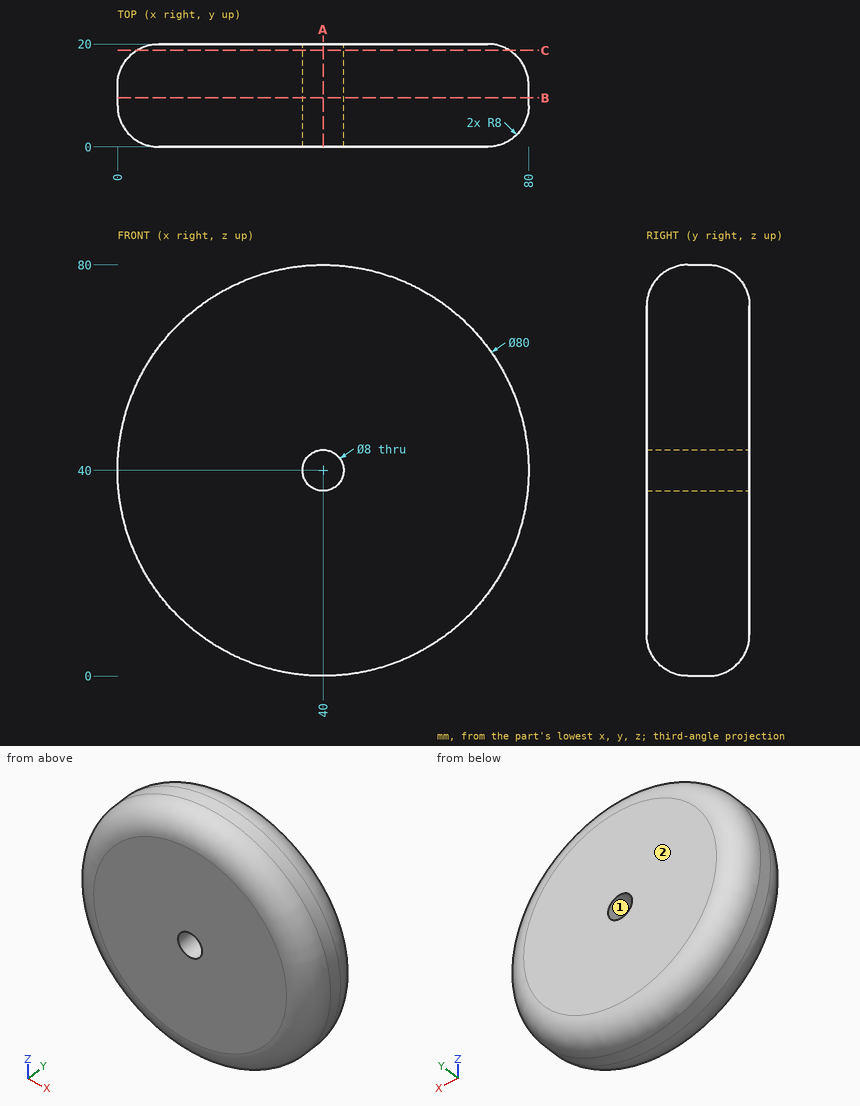
Geometry: see drawing. Coordinates: mm, zero at the bounding-box minimum. Round coordinates to 2 decimals unless told otherwise and drop trailing zeros. Loops run counter-clockwise (first coordinate to the right, second up) from the corner with the lowest first, then second, coordinate; pieces in that order, holes last. Notation, with made-up numbers: (-34.75, 55) -> (-27.75, 55) arc R22 ccw to (-27.75, 79) -> close; hole circle Ø10 at (64, 5.25). An arc over 180 degrees is marked (long way). Use one line per item in the form item = value. Start each with the question number.
Item 1: Material intervals for L1, parallel to Z at x = 40, y = 9.5; L2, parallel to X at y = 9, z = 64; L3, parallel to X at y = 13.75, z = 6.5, sorted ascending. Write a range as from..to.
Item 2: Section query C-C on y = 18.75. Return the cut outline in (x, z), then the cut area to 3 significant figures.
Item 3: Section query B-B on y = 9.5. Return the cut outline in (x, z), then the cut area to 3 significant figures.
Item 4: Section query A-A on x = 40. Return the cut outline in (y, z).
Item 5: Mould query, pull axis X, two halves, no side actions, for the marked faces 1 and 2. Classes: pulls with the +X half, pulls with the -X half, needs draft (parallel to the pull), parting line crosses it, or undercut.
Item 6: Contact query for flat-ended pins moving along their axis: pin 1 Ø8 at (x, y) = (59, 10.5) entering from +Z; pin 2 Ø5 at (x, y) = (14, 16) entering from -Z; pin 3 Ø1.5 at (y, z) = (5.5, 18) entering from -X. Output: stop coordinate, or through.
Ans:
q1.L1 = 0..36, 44..80
q1.L2 = 8..72
q1.L3 = 18.5..61.5
q2.outline = circle Ø72.59 at (40, 40); hole circle Ø8 at (40, 40)
q2.area = 4,090 mm^2
q3.outline = circle Ø80 at (40, 40); hole circle Ø8 at (40, 40)
q3.area = 4,980 mm^2
q4.outline = (0, 8) arc R8 ccw to (8, 0) -> (12, 0) arc R8 ccw to (20, 8) -> (20, 36) -> (0, 36) -> close; (0, 44) -> (20, 44) -> (20, 72) arc R8 ccw to (12, 80) -> (8, 80) arc R8 ccw to (0, 72) -> close
q5.face_1 = undercut
q5.face_2 = needs draft
q6.pin_1 = 77.08
q6.pin_2 = 8.49
q6.pin_3 = 6.51
